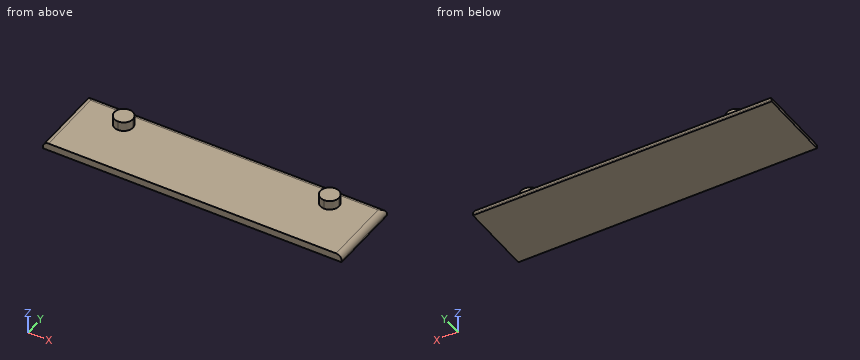
from build123d import *

# Parameters (mm, degrees)
F0_W     = 101.6
F0_H     = 25.4
F1_DEPTH = 2.54
F2_R     = 1.905
F4_DEPTH = 3.175


with BuildPart() as f1:
    # F0 (on Top) → F1 (new body)
    with BuildSketch(Plane.XY):
        with Locations((34.925, 0)):
            Rectangle(F0_W, F0_H)
        with BuildLine():
            Line((69.85, 0), (0, 0))
            Line((0, 0), (0, 3.175))
            ThreePointArc((0, 3.175), (-2.2450640303, 8.5950640303), (3.175, 6.35))
            Line((3.175, 6.35), (66.675, 6.35))
            ThreePointArc((66.675, 6.35), (69.85, 9.525), (73.025, 6.35))
            ThreePointArc((73.025, 6.35), (72.0950640303, 4.1049359697), (69.85, 3.175))
            Line((69.85, 3.175), (69.85, 0))
        make_face(mode=Mode.SUBTRACT)
        with BuildLine():
            Line((0, 3.175), (0, 0))
            Line((0, 0), (69.85, 0))
            Line((69.85, 0), (69.85, 3.175))
            ThreePointArc((69.85, 3.175), (67.6049359697, 4.1049359697), (66.675, 6.35))
            Line((66.675, 6.35), (3.175, 6.35))
            ThreePointArc((3.175, 6.35), (2.2450640303, 4.1049359697), (0, 3.175))
        make_face()
        with BuildLine():
            Line((69.85, 6.35), (69.85, 3.175))
            ThreePointArc((69.85, 3.175), (72.0950640303, 4.1049359697), (73.025, 6.35))
            ThreePointArc((73.025, 6.35), (69.85, 9.525), (66.675, 6.35))
            Line((66.675, 6.35), (69.85, 6.35))
        make_face()
        with BuildLine():
            ThreePointArc((3.175, 6.35), (-2.2450640303, 8.5950640303), (0, 3.175))
            Line((0, 3.175), (0, 6.35))
            Line((0, 6.35), (3.175, 6.35))
        make_face()
        with BuildLine():
            Line((0, 6.35), (0, 3.175))
            ThreePointArc((0, 3.175), (2.2450640303, 4.1049359697), (3.175, 6.35))
            Line((3.175, 6.35), (0, 6.35))
        make_face()
        with BuildLine():
            ThreePointArc((66.675, 6.35), (67.6049359697, 4.1049359697), (69.85, 3.175))
            Line((69.85, 3.175), (69.85, 6.35))
            Line((69.85, 6.35), (66.675, 6.35))
        make_face()
    extrude(amount=F1_DEPTH)

    # F2
    f2_edges = [f1.edges().sort_by_distance(p)[0] for p in [
        (34.925, 12.7, 2.54),
        (-15.875, 0, 2.54),
        (85.725, 0, 2.54),
    ]]
    fillet(f2_edges, radius=F2_R)

    # F3 (on face) → F4 (join)
    with BuildSketch(Plane.XY.offset(2.54)):
        with BuildLine():
            ThreePointArc((66.939, 6.35), (67.8660070375, 4.1120070375), (70.104, 3.185))
            Line((70.104, 3.185), (70.104, 6.35))
            Line((70.104, 6.35), (66.939, 6.35))
        make_face()
        with BuildLine():
            Line((70.104, 6.35), (70.104, 3.185))
            ThreePointArc((70.104, 3.185), (72.3419929625, 4.1120070375), (73.269, 6.35))
            ThreePointArc((73.269, 6.35), (70.104, 9.515), (66.939, 6.35))
            Line((66.939, 6.35), (70.104, 6.35))
        make_face()
        with BuildLine():
            Line((0, 6.35), (0, 3.185))
            ThreePointArc((0, 3.185), (2.2379929625, 4.1120070375), (3.165, 6.35))
            Line((3.165, 6.35), (0, 6.35))
        make_face()
        with BuildLine():
            ThreePointArc((3.165, 6.35), (-2.2379929625, 8.5879929625), (0, 3.185))
            Line((0, 3.185), (0, 6.35))
            Line((0, 6.35), (3.165, 6.35))
        make_face()
    extrude(amount=F4_DEPTH)


solid = f1.part
Work out the finished part from the listing and answer in its coordinate system (mm). Round coordinates to 2 decimals unless told otherwise and drop trailing zeros. Order: outer loops, then holes, each group sorted by start corner. A loop starts at its lowest first (then second) coordinate and runs counter-clockwise, first axis right, second up. Notation, with made-up numbers: M 5,84.5 L 35,84.5 A9 cw 35,94.5 Z; hole C 64.5,-21 d6. An arc over 180 degrees is marked long. Put each result on its own line as item: value. Start each with the question number.
Q1. Flat-ended cylindrical pins translate along their axes: pin 1 (1.5 mm diameter, centred on y = 1.5, z = 4, fed in from +X); pin 2 (7 mm diameter, centred on x = 38.5, y = -5, fed in from +Z). Find the tip coordinate at first contact, or state that the pin passes through.
Q2. Section B-B, the plane x = 77.5 is taken. Write down the section's boundary in (y, z) (3 decimals).
Q3. Section A-A, the plane z = 4.6 is taken. Write down the section's boundary in (x, y) (3 decimals), and give its area (3 significant figures).
Q4. Section C-C, the plane y = -6 is taken. Write down the section's boundary in (x, z) (3 decimals).
Q5. Straight lines are drawn through the part: L1, parallel to Z at x = 18, y = -7; L2, parallel to X at y = 4, z = 3.2; L3, parallel to X at y = 7.5, z = 4.4. For each, find the intervals that lie inside material, in ascending order. Write a range as [from, to].
Findings below:
1. pin 1: passes through
1. pin 2: stops at z = 2.54
2. outline: M -12.7,0 L 12.7,0 L 12.7,0.635 A1.905 ccw 10.795,2.54 L -12.7,2.54 Z
3. outline: C 0,6.35 d6.33; C 70.104,6.35 d6.33
3. area: 62.9 mm^2
4. outline: M -15.875,0 L 85.725,0 L 85.725,0.635 A1.905 ccw 83.82,2.54 L -13.97,2.54 A1.905 ccw -15.875,0.635 Z
5. L1: z = [0, 2.54]
5. L2: x = [-2.12, 2.12], [67.98, 72.22]
5. L3: x = [-2.95, 2.95], [67.16, 73.05]
